```python
from build123d import *

# Parameters (mm, degrees)
SKETCH_1_W          = 700
SKETCH_1_H          = 300
EXTRUDE_1_DEPTH     = 500
FILLET_1_R          = 10
SKETCH_2_W          = 650.999625187
SKETCH_2_H          = 106.196586902
SKETCH_2_H_2        = 130.199925037
CUT_EXTRUDE_1_DEPTH = 280


with BuildPart() as part:
    # 草图1 → 凸台-拉伸1 (new body)
    with BuildSketch(Plane(origin=(0, 0, 0), x_dir=(1, 0, 0), z_dir=(0, 1, 0))):
        Rectangle(SKETCH_1_W, SKETCH_1_H)
    extrude(amount=EXTRUDE_1_DEPTH)

    # 圆角1
    fillet_1_edges = [part.edges().sort_by_distance(p)[0] for p in [
        (350, 500, 0),
        (0, 500, -150),
        (-350, 500, 0),
        (0, 0, -150),
        (350, 0, 0),
        (0, 0, 150),
        (-350, 0, 0),
        (0, 500, 150),
        (-350, 250, -150),
        (350, 250, -150),
        (350, 250, 150),
        (-350, 250, 150),
    ]]
    fillet(fillet_1_edges, radius=FILLET_1_R)

    # 草图2 → 切除-拉伸1 (cut)
    with BuildSketch(Plane(origin=(0, 0, -150), x_dir=(-1, 0, 0), z_dir=(0, 0, -1))):
        with Locations((2.909495531, 414.750184475)):
            Rectangle(SKETCH_2_W, SKETCH_2_H)
        with Locations((2.909495531, 185.263724423)):
            Rectangle(SKETCH_2_W, SKETCH_2_H_2)
    extrude(amount=-CUT_EXTRUDE_1_DEPTH, mode=Mode.SUBTRACT)


solid = part.part
```
The listing builds one solid part. Answer for the finished solid, in the listing's coordinates (mm). A direction names the side the tool comes from. Round coordinates to 2 decimals unless told otherwise and drop trailing zeros. Loops run counter-clockwise (first coordinate to the right, second up) from the corner with the lowest first, then second, coordinate; pieces in that order, holes last. Notation, with made-up numbers: (63.25, 55.5) - (111.25, 55.5) arc R20 cw to (111.25, 82.5) - close; hole circle Ø11 at (-19.5, 34). An arc over 180 degrees is marked (long way). Use one line per item in the form item = value. Start each with the question number.
1. For a pull along X with two mould halves and no side action, classify faces 3 (the face through (-5, 0, -2)), 4 (the face through (2, 120.164, -12)), 5 (the face through (350, 247, 2)) as pulls with the +X half, pulls with the -X half, needs draft (parallel to the pull), parting line crosses it, or undercut.
2. The part is cut by section C-C on y = 143. Determine the outline of the cut face in (x, z).
3. The part is cut by section B-B on x = 117. Determine the outline of the cut face in (y, z).
4. Consider line 1 (Y direction, x = -191, z = -27.5); line 2 (X direction, y = 141, z = 92); line 3 (Z direction, x = 81, y = 424). Determine where each line is inside the solid, lowest interval first. Write a range as [from, to].
5. A tool of negligible diameter and unlimited length cuts with its end or side. For faces 1 (the face through (2, 415, 130)), 2 (the face through (-350, 247, 2)), from which of +Z, -Z, +X, -X, +Y, -Y can it reach the whole face along a straight path? Write none if from no direction.
6. The part is cut by section A-A on z = 99. Determine the outline of the cut face in (x, y), then the cut area to 3 significant figures.
Geometry check:
q1.face_3 = needs draft
q1.face_4 = undercut
q1.face_5 = pulls with the +X half
q2.outline = (-350, -140) arc R10 ccw to (-340, -150) - (-328.41, -150) - (-328.41, 130) - (322.59, 130) - (322.59, -150) - (340, -150) arc R10 ccw to (350, -140) - (350, 140) arc R10 ccw to (340, 150) - (-340, 150) arc R10 ccw to (-350, 140) - close
q3.outline = (0, -140) arc R10 ccw to (10, -150) - (120.16, -150) - (120.16, 130) - (250.36, 130) - (250.36, -150) - (361.65, -150) - (361.65, 130) - (467.85, 130) - (467.85, -150) - (490, -150) arc R10 ccw to (500, -140) - (500, 140) arc R10 ccw to (490, 150) - (10, 150) arc R10 ccw to (0, 140) - close
q4.line_1 = [0, 120.16], [250.36, 361.65], [467.85, 500]
q4.line_2 = [-350, -328.41], [322.59, 350]
q4.line_3 = [130, 150]
q5.face_1 = -Z
q5.face_2 = +Z, -Z, -X, +Y, -Y
q6.outline = (-350, 10) arc R10 ccw to (-340, 0) - (340, 0) arc R10 ccw to (350, 10) - (350, 490) arc R10 ccw to (340, 500) - (-340, 500) arc R10 ccw to (-350, 490) - close; hole (-328.41, 120.16) - (322.59, 120.16) - (322.59, 250.36) - (-328.41, 250.36) - close; hole (-328.41, 361.65) - (322.59, 361.65) - (322.59, 467.85) - (-328.41, 467.85) - close
q6.area = 196,000 mm^2
